Check sheet for the modelled part. Datum: model origin and axes. Units: mm. Face numbers are marked on the shaded views. A direction names the side the tool comes from. Give positions to 0.01 mm unless a question says otherwise; leave off trailing zeros. Order: outer loops, then holes, each group sorted by start corner. A loop starts at its lowest first (then second) coordinate and runs counter-clockwise, first axis right, second up.
from build123d import *

# Parameters (mm, degrees)
F1_DEPTH = 25.4


with BuildPart() as f1:
    # F0 (on Top) → F1 (new body)
    with BuildSketch(Plane.XY):
        Polygon((-11.13816, -15.454575), (-27.68127, -38.1), (0, -19.05), (27.68127, -38.1), (11.13816, -15.454575), (44.789236, 14.552905), (12.292903, 14.552905), (0, 47.09419), (-12.292903, 14.552905), (-44.789236, 14.552905), align=None)
        Polygon((-36.458193, 11.377905), (-10.098309, 11.377905), (0, 38.109749), (10.098309, 11.377905), (36.458193, 11.377905), (6.875413, -15.001777), (14.111704, -24.907345), (0, -15.195797), (-14.111704, -24.907345), (-6.875413, -15.001777), align=None, mode=Mode.SUBTRACT)
    extrude(amount=F1_DEPTH)


solid = f1.part
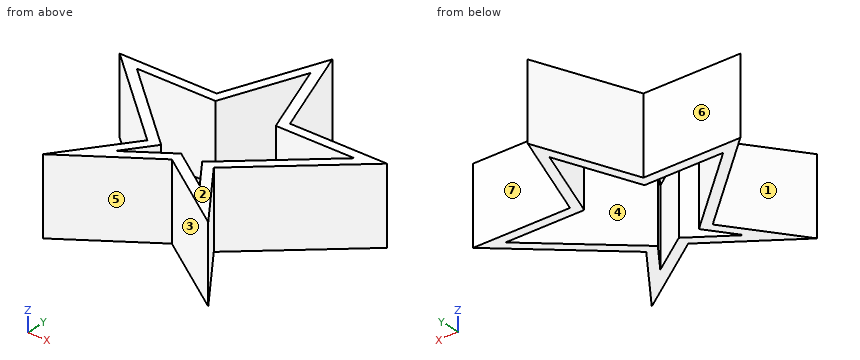
1) Section check C-C, the plane y = 21.5. Record the cut outline in (x, z).
Recorded:
outline: (-9.67, 0) - (-6.27, 0) - (-6.27, 25.4) - (-9.67, 25.4) - close; (6.27, 0) - (9.67, 0) - (9.67, 25.4) - (6.27, 25.4) - close
2) Material ranges on L1, parallel to X at y = -17.5, z = 16; L2, parallel to X at y = -15.5, z = 17.25; L3, parallel to X at y = -24.5, z = 13.5, recorded low to high.
Recorded:
L1: x = -12.63 to -8.7, -3.35 to 3.35, 8.7 to 12.63
L2: x = -11.17 to -7.24, -0.44 to 0.44, 7.24 to 11.17
L3: x = -17.75 to -13.81, -13.52 to -7.92, 7.92 to 13.52, 13.81 to 17.75
3) Section check D-D, the plane x = 29. Record the cut outline in (y, z), then the cut area to 3 significant figures.
Recorded:
outline: (0.47, 0) - (4.73, 0) - (4.73, 25.4) - (0.47, 25.4) - close; (11.38, 0) - (14.55, 0) - (14.55, 25.4) - (11.38, 25.4) - close
area: 189 mm2
4) Section check A-A, the plane z = 4. Record the cut outline in (x, y).
Recorded:
outline: (-44.79, 14.55) - (-11.14, -15.45) - (-27.68, -38.1) - (0, -19.05) - (27.68, -38.1) - (11.14, -15.45) - (44.79, 14.55) - (12.29, 14.55) - (0, 47.09) - (-12.29, 14.55) - close; hole (-36.46, 11.38) - (-6.88, -15) - (-14.11, -24.91) - (0, -15.2) - (14.11, -24.91) - (6.88, -15) - (36.46, 11.38) - (10.1, 11.38) - (0, 38.11) - (-10.1, 11.38) - close
5) Section check B-B, the plane x = -26.5. Record the cut outline in (y, z).
Recorded:
outline: (-37.29, 0) - (-36.48, 0) - (-36.48, 25.4) - (-37.29, 25.4) - close; (-1.76, 0) - (2.5, 0) - (2.5, 25.4) - (-1.76, 25.4) - close; (11.38, 0) - (14.55, 0) - (14.55, 25.4) - (11.38, 25.4) - close
6) Set-up check for the marked faces 4, 5, 6 and 7: record each of +Z, -Z, +X, -X, +Y, -Y from which the full face is reachable in a straight line by a thin tool's end or side.
Recorded:
face 4: +Z, -Z
face 5: +Z, -Z, -Y
face 6: +Z, -Z, -X, +Y
face 7: +Z, -Z, +X, +Y
7) Depth check by flat-ended pin: pin 1 Ø8 at (y, z) = (-3, 5) entering from -X; pin 2 Ø10 at (y, z) = (29.5, 5.5) entering from +X; pin 3 Ø8 at (y, z) = (26, 22.5) entering from -X. Enter the tip coordinate at first touch or a pass-through.
Recorded:
pin 1: stops at x = -29.59
pin 2: stops at x = 8.54
pin 3: stops at x = -9.48
8) Draft check along Y on the marked faces 1, 2 and 3. Enter one of: +Y half, -Y half, draft (parallel to the pull), parting line (faces both ways), or undercut.
Recorded:
face 1: undercut
face 2: draft
face 3: -Y half
